For this review, use the dimensioned drawing (mm, ordinates from the lowest corner) and the shaded views. Give positions to 0.01 mm unless a question says otherwise; leave off trailing zeros. Write each loop counter-clockwise with the first axis right and the second up, starting at its lowest first coordinate (ties: lowest second). Pieces come first, ordered by that corner, then holes. Notation, with made-up numbers: M 45,73.5 L 102,73.5 A11 cw 102,90.5 Z; hole C -18,52.5 d10. An arc over 180 degrees is marked long. Use a Markdown table: item, result. Add a question column.
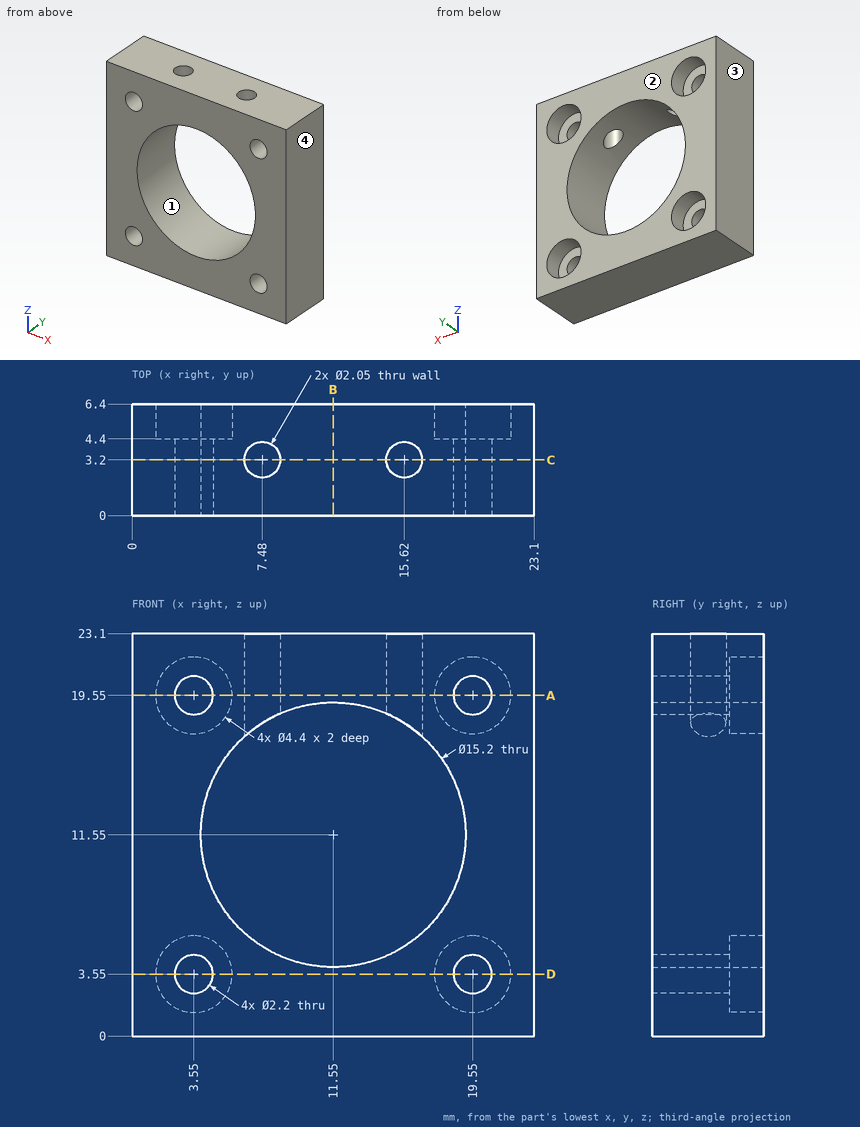
(1) Wall thickness on L1, parallel to X at y = 0.9, z = 3.55; L2, parallel to X at y = 5.5, z = 3.55: over which ranges is each line inside the solid? List them lowest first.
(2) Add section B-B on x = 11.55. Give the boundary of the cut face in (y, z), then the cut area to 3 significant figures.
(3) Add section D-D on z = 3.55. Give the boundary of the cut face in (x, y), then the cut area to 3 significant figures.
(4) Add section A-A on z = 19.55. Give the boundary of the cut face in (x, y) (3 decimals).
(5) Add section C-C on y = 3.2. Give the boundary of the cut face in (x, z) (3 decimals).
(6) The part is to be moulded in two halves that separate along X. For the marked faces 1, 2, 3 and 4, say which applies: released by +X, released by -X, zero draft, split by the parting line, or undercut.
(7) For pin 1 (1.8 mm diameter, centred on x = 19.55, z = 19.55, fed in from +Y); pin 2 (1 mm diameter, centred on y = 6, z = 7, fed in from -X); pin 3 (2 mm diameter, centred on x = 3, z = 4, fed in from +Y), all flat-tipped, find the tip position at first contact; note any pin that passes through.
From the geometry:
| question | item | result |
|---|---|---|
| 1 | L1 | x = 0 to 2.45, 4.65 to 18.45, 20.65 to 23.1 |
| 1 | L2 | x = 0 to 1.35, 5.75 to 17.35, 21.75 to 23.1 |
| 2 | outline | M 0,0 L 6.4,0 L 6.4,3.95 L 0,3.95 Z; M 0,19.15 L 6.4,19.15 L 6.4,23.1 L 0,23.1 Z |
| 2 | area | 50.6 mm^2 |
| 3 | outline | M 0,0 L 2.45,0 L 2.45,4.4 L 1.35,4.4 L 1.35,6.4 L 0,6.4 Z; M 4.65,0 L 18.45,0 L 18.45,4.4 L 17.35,4.4 L 17.35,6.4 L 5.75,6.4 L 5.75,4.4 L 4.65,4.4 Z; M 20.65,0 L 23.1,0 L 23.1,6.4 L 21.75,6.4 L 21.75,4.4 L 20.65,4.4 Z |
| 3 | area | 111 mm^2 |
| 4 | outline | M 0,0 L 2.45,0 L 2.45,4.4 L 1.35,4.4 L 1.35,6.4 L 0,6.4 Z; M 4.65,0 L 18.45,0 L 18.45,4.4 L 17.35,4.4 L 17.35,6.4 L 5.75,6.4 L 5.75,4.4 L 4.65,4.4 Z; M 20.65,0 L 23.1,0 L 23.1,6.4 L 21.75,6.4 L 21.75,4.4 L 20.65,4.4 Z; hole C 7.48,3.2 d2.05; hole C 15.62,3.2 d2.05 |
| 5 | outline | M 0,0 L 23.1,0 L 23.1,23.1 L 16.645,23.1 L 16.645,17.189 A7.6 cw long 6.455,17.189 L 6.455,23.1 L 0,23.1 Z; M 8.505,18.513 A7.6 cw 14.595,18.513 L 14.595,23.1 L 8.505,23.1 Z; hole C 3.55,3.55 d2.2; hole C 3.55,19.55 d2.2; hole C 19.55,3.55 d2.2; hole C 19.55,19.55 d2.2 |
| 6 | face 1 | undercut |
| 6 | face 2 | zero draft |
| 6 | face 3 | released by -X |
| 6 | face 4 | released by +X |
| 7 | pin 1 | passes through |
| 7 | pin 2 | stops at x = 0 |
| 7 | pin 3 | stops at y = 4.4 |
